```python
from build123d import *

# Parameters (mm, degrees)
SZKIC1_R                    = 2
DODANIE_WYCI_GNI_CIE1_DEPTH = 81
DODANIE_WYCI_GNI_CIE2_DEPTH = 3
SZKIC3_R                    = 2.5
DODANIE_WYCI_GNI_CIE3_DEPTH = 19


with BuildPart() as part:
    # Szkic1 → Dodanie-wyciągnięcie1 (new body)
    with BuildSketch(Plane(origin=(0, 0, 0), x_dir=(1, 0, 0), z_dir=(0, 1, 0))):
        Polygon((6, 0), (36, 0), (42, 6), (42, 36), (36, 42), (6, 42), (0, 36), (0, 6), align=None)
        with Locations(Location((33.727922061, 33.727922061, 0), (0, 0, 270))):
            Circle(SZKIC1_R, mode=Mode.SUBTRACT)
        with Locations(Location((33.727922061, 8.272077939, 0), (0, 0, 270))):
            Circle(SZKIC1_R, mode=Mode.SUBTRACT)
        with Locations(Location((8.272077939, 8.272077939, 0), (0, 0, 270))):
            Circle(SZKIC1_R, mode=Mode.SUBTRACT)
        with Locations(Location((8.272077939, 33.727922061, 0), (0, 0, 270))):
            Circle(SZKIC1_R, mode=Mode.SUBTRACT)
    extrude(amount=DODANIE_WYCI_GNI_CIE1_DEPTH)

    # Szkic2 → Dodanie-wyciągnięcie2 (add)
    with BuildSketch(Plane(origin=(0, 81, 0), x_dir=(1, 0, 0), z_dir=(0, 1, 0))):
        with BuildLine():
            ThreePointArc((33.5, 21), (29.838834765, 29.838834765), (21, 33.5))
            Line((21, 33.5), (21, 21))
            Line((21, 21), (33.5, 21))
        make_face()
        with BuildLine():
            Line((21, 21), (21, 33.5))
            ThreePointArc((21, 33.5), (12.161165235, 12.161165235), (33.5, 21))
            Line((33.5, 21), (21, 21))
        make_face()
    extrude(amount=DODANIE_WYCI_GNI_CIE2_DEPTH)

    # Szkic3 → Dodanie-wyciągnięcie3 (add)
    with BuildSketch(Plane(origin=(0, 84, 0), x_dir=(1, 0, 0), z_dir=(0, 1, 0))):
        with Locations(Location((21, 21, 0), (0, 0, 270))):
            Circle(SZKIC3_R)
    extrude(amount=DODANIE_WYCI_GNI_CIE3_DEPTH)


solid = part.part
```
Build history of the part. All positions in model axes, mm. A direction names the side the tool comes from. Round coordinates to 2 decimals unless told otherwise and drop trailing zeros. Order: outer loops, then holes, each group sorted by start corner. A loop starts at its lowest first (then second) coordinate and runs counter-clockwise, first axis right, second up. Notation, with made-up numbers: (29.25, 64) - (44.25, 64) arc R28 cw to (44.25, 102) - close; hole circle Ø2 at (-39, 19). An arc over 180 degrees is marked (long way). Use a Markdown table: item, result.
1) Saw through at A-A on y = 49.5. Write the cut outline in (x, z).
Recorded:
| item | result |
|---|---|
| outline | (0, -36) - (6, -42) - (36, -42) - (42, -36) - (42, -6) - (36, 0) - (6, 0) - (0, -6) - close; hole circle Ø4 at (8.27, -33.73); hole circle Ø4 at (8.27, -8.27); hole circle Ø4 at (33.73, -33.73); hole circle Ø4 at (33.73, -8.27) |
2) Saw through at D-D on x = 39.5. Write the cut outline in (y, z), and give its area (4 significant figures).
Recorded:
| item | result |
|---|---|
| outline | (0, -38.5) - (81, -38.5) - (81, -3.5) - (0, -3.5) - close |
| area | 2,835 mm² |
3) Flat gauge pins, fed straight in: pin 1 Ø4 at (x, y) = (22.5, 66.5) entering from +Z; pin 2 Ø6.5 at (x, z) = (8.27, -8.27) entering from +Y; pin 3 Ø7.5 at (x, z) = (15.5, -25) entering from +Y. Where does each tip first touch, or does it go through?
Recorded:
| item | result |
|---|---|
| pin 1 | stops at z = 0 |
| pin 2 | stops at y = 81 |
| pin 3 | stops at y = 84 |
4) Tool access for faces 1 (the face through (11, 81, -31)), 2 (the face through (0, 40, -21)): list every direction of +Z, -Z, +X, -X, +Y, -Y with a clear straight run to the whole face (end or side of a thin tool).
Recorded:
| item | result |
|---|---|
| face 1 | +Y |
| face 2 | +Z, -Z, -X, +Y, -Y |
5) Saw through at B-B on x = 14. Write the cut outline in (y, z).
Recorded:
| item | result |
|---|---|
| outline | (0, -42) - (81, -42) - (81, -31.36) - (84, -31.36) - (84, -10.64) - (81, -10.64) - (81, 0) - (0, 0) - close |
6) Saw through at C-C on z = -30. Write the cut outline in (x, y).
Recorded:
| item | result |
|---|---|
| outline | (0, 0) - (42, 0) - (42, 81) - (29.67, 81) - (29.67, 84) - (12.33, 84) - (12.33, 81) - (0, 81) - close |
7) Wall check: L1, parallel to X at y = 62, z = -6.5; L2, parallel to X at y = 47.5, z = -7.5; L3, parallel to Z at x = 7, y = 12. Give the ranges that are in metal, low to high.
Recorded:
| item | result |
|---|---|
| L1 | x = 0 to 7.34, 9.2 to 32.8, 34.66 to 42 |
| L2 | x = 0 to 6.43, 10.12 to 31.88, 35.57 to 42 |
| L3 | z = -42 to -35.27, -32.18 to -9.82, -6.73 to 0 |
8) Pull direction Z, two halves, no side cores. Call faces 3 (the face through (8.36, 39.933, -35.726)), 4 (the face through (8.873, 39.933, -6.364)), 5 (the face through (42, 40, -21)), 6 (the face through (3, 40, -3)): pulls with the +Z half, pulls with the -Z half, needs draft (parallel to the pull), parting line crosses it, or undercut.
Recorded:
| item | result |
|---|---|
| face 3 | undercut |
| face 4 | undercut |
| face 5 | needs draft |
| face 6 | pulls with the +Z half |
